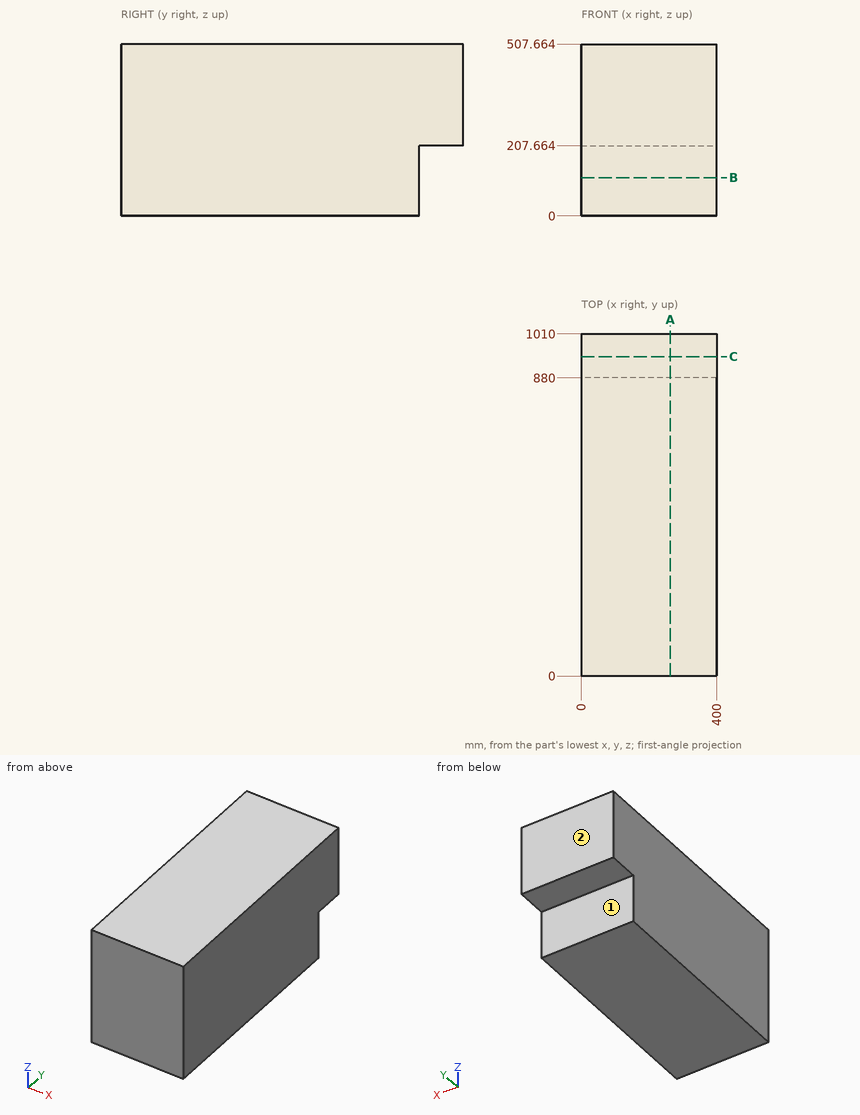
Can you work these out from the drawing? Everything is in mm from the part's minimum corner. A direction names the side the tool comes from. Give positions to 0.01 mm unless a question says otherwise; leave off trailing zeros. Order: outer loops, then holes, each group sorted by start corner. A loop starts at its lowest first (then second) coordinate and runs counter-clockwise, first axis right, second up.
1. I need wall thicknesses on L1, parallel to Y at x = 29, z = 187; L2, parallel to Z at x = 351, y = 946. Which ranges of each line are inside material? Lowest first, please.
2. Suppose I cut it at B-B (z = 113). List the corners of the cut face in (x, y) for me, plus the area to 3 significant figures.
3. Will this pin go through, and if not, where does the flat tip stop? P1, Ø3, axis at x = 297, z = 198, coming from the +Y side.
4. Suppose I cut it at C-C (y = 943). List the corners of the cut face in (x, z) for me, plus the area to 3 significant figures.
5. For the marked faces 1 and 2, which set-ups out of +Z, -Z, +X, -X, +Y, -Y let a thin tool reach every point of the face, with its end or its side?
6. Suppose I cut it at A-A (x = 263). List the corners of the cut face in (y, z) for me.
Solved:
1. L1: y = 0 to 880
1. L2: z = 207.66 to 507.66
2. outline: (0, 0) - (400, 0) - (400, 880) - (0, 880) - close
2. area: 352,000 mm2
3. P1: stops at y = 880
4. outline: (0, 207.66) - (400, 207.66) - (400, 507.66) - (0, 507.66) - close
4. area: 120,000 mm2
5. face 1: -Z, +X, -X, +Y
5. face 2: +Z, -Z, +X, -X, +Y
6. outline: (0, 0) - (880, 0) - (880, 207.66) - (1010, 207.66) - (1010, 507.66) - (0, 507.66) - close
